CAD build for the part. Positions are in the model's coordinates, mm. A direction names the side the tool comes from. Give positions to 0.01 mm unless a question says otherwise; leave off trailing zeros. Loops run counter-clockwise (first coordinate to the right, second up) from the corner with the lowest first, then second, coordinate; pieces in that order, holes last.
Item 1: Mould opens along X. For faces 1 (the cylindrical face through (-1.08, -4.88, 2.47)), 2 (the cylindrical face through (0.209, 9.523, 31.595)), 3 (the flat face through (0, -10, 17)), 4 (the cylindrical face through (1.154, -12.465, 25.283)) say: released by +X, released by -X, zero draft, split by the parting line, or undercut.
Item 2: Saw through at D-D on y = -11.75. Give the cut face in (x, z) (3 decimals), plus the area to 3 significant figures.
Item 3: Saw through at C-C on x = -4.25. Give the cut face in (y, z).
Item 4: Saw through at A-A on x = 0. Give the cut face in (y, z) (3 decimals), plus the area to 3 significant figures.
Item 5: Probe probe 1 along Z at (x, y) = (0, -11.3) (3 decimals); probe 2 along Y at (x, z) = (0, 32.45) (3 decimals); probe 3 along Z at (x, y) = (1.25, -7). List the from-to ranges inside material, lowest first.
Item 6: Which spindle directions (+Z, -Z, +X, -X, +Y, -Y) get a long thin tool onto all of the face, cutting with end or side? Do faces 5 (the flat face through (2, -5, 29.13)), 6 (the flat face through (-9.525, -11, 17)). Say none if no direction does.
Item 7: Drop flat-ended pins along their axis: P1, Ø6.5, axis at x = 0, z = 11.065, coming from the +Y side; P2, Ø6.5, axis at x = 0, z = 23.065, coming from the -Y side. Give the stop position or say it passes through.
Item 8: Saw through at B-B on y = -0.5. Give the cut face in (x, z) (3 decimals).
from build123d import *

# Parameters (mm, degrees)
SKETCH1_R           = 9.525
SKETCH1_R_2         = 5
BOSS_EXTRUDE1_DEPTH = 34.13
SKETCH2_W           = 24.13
SKETCH2_H           = 19.525
CUT_EXTRUDE1_DEPTH  = 42.865969474
SKETCH3_R           = 2.5
CUT_EXTRUDE2_DEPTH  = 41.45748571


with BuildPart() as part:
    # Sketch1 → Boss-Extrude1 (new body)
    # profile 1 of 2: a face of its own
    with BuildSketch(Plane.XY):
        Circle(SKETCH1_R)
        Circle(SKETCH1_R_2, mode=Mode.SUBTRACT)
    # profile 2 of 2: a face of its own
    with BuildSketch(Plane.XY):
        with BuildLine():
            ThreePointArc((9.525, 0), (0, -9.525), (-9.525, 0))
            Line((-9.525, 0), (-9.525, -15))
            Line((-9.525, -15), (9.525, -15))
            Line((9.525, -15), (9.525, 0))
        make_face()
    extrude(amount=BOSS_EXTRUDE1_DEPTH)

    # Sketch2 → Cut-Extrude1 (cut, through all)
    with BuildSketch(Plane(origin=(9.525, 0, 0), x_dir=(0, 0, -1), z_dir=(1, 0, 0))):
        with Locations((-17.065, -0.2375)):
            Rectangle(SKETCH2_W, SKETCH2_H)
    extrude(amount=-CUT_EXTRUDE1_DEPTH, mode=Mode.SUBTRACT)

    # Sketch3 → Cut-Extrude2 (cut, through all)
    with BuildSketch(Plane(origin=(0, -10, 0), x_dir=(1, 0, 0), z_dir=(0, 1, 0))):
        with Locations(Location((0, -11.065, 0), (0, 0, 180))):
            Circle(SKETCH3_R)
        with Locations((0, -23.065)):
            Circle(SKETCH3_R)
    extrude(amount=-CUT_EXTRUDE2_DEPTH, mode=Mode.SUBTRACT)


solid = part.part
Results below:
1. face 1: undercut
1. face 2: split by the parting line
1. face 3: zero draft
1. face 4: undercut
2. outline: (-9.525, 0) - (9.525, 0) - (9.525, 34.13) - (-9.525, 34.13) - close; hole circle Ø5 at (0, 11.065); hole circle Ø5 at (0, 23.065)
2. area: 611 mm2
3. outline: (-15, 0) - (-2.63, 0) - (-2.63, 5) - (-10, 5) - (-10, 29.13) - (-2.63, 29.13) - (-2.63, 34.13) - (-15, 34.13) - close; (2.63, 0) - (8.52, 0) - (8.52, 5) - (2.63, 5) - close; (2.63, 29.13) - (8.52, 29.13) - (8.52, 34.13) - (2.63, 34.13) - close
4. outline: (-15, 0) - (-5, 0) - (-5, 5) - (-10, 5) - (-10, 8.565) - (-15, 8.565) - close; (-15, 13.565) - (-10, 13.565) - (-10, 20.565) - (-15, 20.565) - close; (-15, 25.565) - (-10, 25.565) - (-10, 29.13) - (-5, 29.13) - (-5, 34.13) - (-15, 34.13) - close; (5, 0) - (9.525, 0) - (9.525, 5) - (5, 5) - close; (5, 29.13) - (9.525, 29.13) - (9.525, 34.13) - (5, 34.13) - close
4. area: 216 mm2
5. probe 1: z = 0 to 8.565, 13.565 to 20.565, 25.565 to 34.13
5. probe 2: y = -15 to -5, 5 to 9.525
5. probe 3: z = 0 to 5, 29.13 to 34.13
6. face 5: +X, -X, +Y
6. face 6: +Z, -Z, -X, +Y, -Y
7. P1: stops at y = -10
7. P2: stops at y = -15
8. outline: (-9.525, 0) - (-4.975, 0) - (-4.975, 5) - (-9.525, 5) - close; (-9.525, 29.13) - (-4.975, 29.13) - (-4.975, 34.13) - (-9.525, 34.13) - close; (4.975, 0) - (9.525, 0) - (9.525, 5) - (4.975, 5) - close; (4.975, 29.13) - (9.525, 29.13) - (9.525, 34.13) - (4.975, 34.13) - close
